```python
from build123d import *

# Parameters (mm, degrees)
F0_W     = 170.18
F0_H     = 87.63
F1_DEPTH = 3.9878
F3_D     = 3


with BuildPart() as f1:
    # F0 (on Front) → F1 (new body)
    with BuildSketch(Plane.XZ):
        with BuildLine():
            Line((90.146613, 65.525748), (-87.653387, 65.525748))
            ThreePointArc((-87.653387, 65.525748), (-96.633644, 61.806004), (-100.353387, 52.825748))
            Line((-100.353387, 52.825748), (-100.353387, -41.154252))
            ThreePointArc((-100.353387, -41.154252), (-96.633644, -50.134508), (-87.653387, -53.854252))
            Line((-87.653387, -53.854252), (90.146613, -53.854252))
            ThreePointArc((90.146613, -53.854252), (99.126869, -50.134508), (102.846613, -41.154252))
            Line((102.846613, -41.154252), (102.846613, 52.825748))
            ThreePointArc((102.846613, 52.825748), (99.126869, 61.806004), (90.146613, 65.525748))
        make_face()
        with Locations((0.491043, 6.588873)):
            Rectangle(F0_W, F0_H, mode=Mode.SUBTRACT)
    extrude(amount=F1_DEPTH)

    # F3 (through all)
    with Locations(Plane.XZ.offset(3.9878)):
        with Locations((-93.95866, 58.1965), (95.760956, 58.250498), (95.760956, -46.399333), (-93.443841, -46.399333)):
            Hole(F3_D / 2)


solid = f1.part
```
Input: part model. Units: mm. Frame: model coordinates. A direction names the side the tool comes from. Round coordinates to 2 decimals unless told otherwise and drop trailing zeros. Loops run counter-clockwise (first coordinate to the right, second up) from the corner with the lowest first, then second, coordinate; pieces in that order, holes last. Notation, with made-up numbers: M 6,-28 L 35,-28 A16 ccw 35,-2 Z; hole C -29.75,41 d7. An arc over 180 degrees is marked long. Answer in a Markdown table with one row per item. Add a question column.
1. Section C-C (y = -2.3). Output: boundary loops of the cut face in (x, z), and give its area (3 significant figures).
2. Section A-A (x = 80.5). Output: boundary loops of the cut face in (y, z).
3. Ray query, probe 1 along X at (y, z) = (-0.7, -22); probe 2 along Z at (x, y) = (64.5, -2.65). Return the intervals inside material, ascending.
4. Section B-B (z = -5.5). Output: boundary loops of the cut face in (x, y), and give its area (3 significant figures).
5. Mould query, pull axis Z, two halves, no side actions, for faces 1 (the face through (0, -2, -53.854)), 2 (the face through (102.847, -2, 5)), 3 (the face through (85.581, -2, 6)). Classes: released by +Z, released by -Z, zero draft, split by the parting line, or undercut.
6. Set-up query: faces 4 (the face through (99.225, -1.966, 61.707)), 5 (the face through (-84.599, -2, 6)). Return all of +Z, -Z, +X, -X, +Y, -Y with unobstructed straight access to the full face (end or side cutting, diameter ignored); none if empty.
7. Contact query for a flat-ended pin moving along its axis: pin 1 (3.5 mm diameter, centred on x = 95.76, z = 58.25, fed in from +Y). Output: stop coordinate, or through.
Values follow:
| question | item | result |
|---|---|---|
| 1 | outline | M -100.35,-41.15 A12.7 ccw -87.65,-53.85 L 90.15,-53.85 A12.7 ccw 102.85,-41.15 L 102.85,52.83 A12.7 ccw 90.15,65.53 L -87.65,65.53 A12.7 ccw -100.35,52.83 Z; hole C -93.96,58.2 d3; hole C -93.44,-46.4 d3; hole M -84.6,-37.23 L 85.58,-37.23 L 85.58,50.4 L -84.6,50.4 Z; hole C 95.76,-46.4 d3; hole C 95.76,58.25 d3 |
| 1 | area | 9,180 mm^2 |
| 2 | outline | M -3.99,-53.85 L 0,-53.85 L 0,-37.23 L -3.99,-37.23 Z; M -3.99,50.4 L 0,50.4 L 0,65.53 L -3.99,65.53 Z |
| 3 | probe 1 | -100.35 to -84.6, 85.58 to 102.85 |
| 3 | probe 2 | -53.85 to -37.23, 50.4 to 65.53 |
| 4 | outline | M -100.35,-3.99 L -84.6,-3.99 L -84.6,0 L -100.35,0 Z; M 85.58,-3.99 L 102.85,-3.99 L 102.85,0 L 85.58,0 Z |
| 4 | area | 132 mm^2 |
| 5 | face 1 | released by -Z |
| 5 | face 2 | zero draft |
| 5 | face 3 | undercut |
| 6 | face 4 | +Z, +X, +Y, -Y |
| 6 | face 5 | +Y, -Y |
| 7 | pin 1 | y = 0 |
